Part model, mm, in its own coordinate system. Face numbers are marked on the shaded views. A direction names the side the tool comes from. Round coordinates to 2 decimals unless told otherwise and drop trailing zeros. Loops run counter-clockwise (first coordinate to the right, second up) from the corner with the lowest first, then second, coordinate; pieces in that order, holes last. Notation, with made-up numbers: (-5, 62) -> (9, 62) arc R15 cw to (9, 83) -> close; hole circle Ø3 at (-19.5, 45). An arc over 180 degrees is marked (long way). Answer as CSV lines item,"result".
from build123d import *

# Parameters (mm, degrees)
F0_W     = 205
F0_H     = 236
F0_R     = 2.25
F0_W_2   = 51
F0_H_2   = 216
F1_DEPTH = 25
F2_W     = 18
F2_H     = 18
F3_DEPTH = 10
F4_R     = 6
F5_DEPTH = 23


with BuildPart() as f1:
    # F0 (on Top) → F1 (new body)
    with BuildSketch(Plane.XY):
        Rectangle(F0_W, F0_H)
        with Locations((-33.5, -54)):
            Circle(F0_R, mode=Mode.SUBTRACT)
        with Locations((33.5, -54)):
            Circle(F0_R, mode=Mode.SUBTRACT)
        with Locations((-67, 0)):
            Rectangle(F0_W_2, F0_H_2, mode=Mode.SUBTRACT)
        with Locations((-33.5, 54)):
            Circle(F0_R, mode=Mode.SUBTRACT)
        Rectangle(F0_W_2, F0_H_2, mode=Mode.SUBTRACT)
        with Locations((33.5, 54)):
            Circle(F0_R, mode=Mode.SUBTRACT)
        with Locations((67, 0)):
            Rectangle(F0_W_2, F0_H_2, mode=Mode.SUBTRACT)
    extrude(amount=F1_DEPTH)

    # F2 (on face) → F3 (cut, through all)
    with BuildSketch(Plane.XZ.offset(118)):
        with Locations((-73.5, 16)):
            Rectangle(F2_W, F2_H)
        with Locations((-6.5, 16)):
            Rectangle(F2_W, F2_H)
        with Locations((60.5, 16)):
            Rectangle(F2_W, F2_H)
    extrude(amount=-F3_DEPTH, mode=Mode.SUBTRACT)

    # F4 (on face) → F5 (cut)
    with BuildSketch(Plane.XY.offset(25)):
        with Locations((-33.5, 54)):
            Circle(F4_R)
        with Locations((-33.5, -54)):
            Circle(F4_R)
        with Locations((33.5, 54)):
            Circle(F4_R)
        with Locations((33.5, -54)):
            Circle(F4_R)
    extrude(amount=-F5_DEPTH, mode=Mode.SUBTRACT)


solid = f1.part
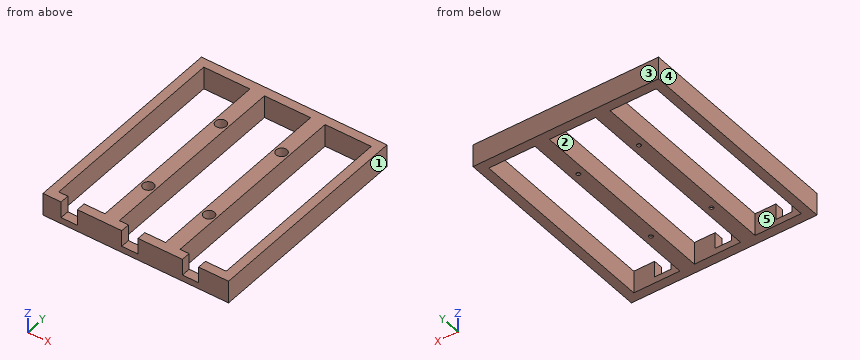
Q1. Saw through at B-B, the plane y = -94. Write the cut outline in (x, z), then the cut area to 3 significant figures.
Geometry results:
outline,"(-102.5, 0) -> (-92.5, 0) -> (-92.5, 25) -> (-102.5, 25) -> close; (-41.5, 0) -> (-25.5, 0) -> (-25.5, 25) -> (-41.5, 25) -> close; (25.5, 0) -> (41.5, 0) -> (41.5, 25) -> (25.5, 25) -> close; (92.5, 0) -> (102.5, 0) -> (102.5, 25) -> (92.5, 25) -> close"
area,"1,300 mm2"
Q2. Saw through at C-C, the plane z = 21.25. Give the number of separate pieces and of enclosed holes in the cut face, then the cut area to 3 significant figures.
Geometry results:
separate pieces,"1"
enclosed holes,"4"
area,"14,300 mm2"
Q3. Two-plate mould, pull along X, no slides. Class the marked faces 1, 2 and 3: pulls with the +X half, pulls with the -X half, needs draft (parallel to the pull), parting line crosses it, or undercut.
Geometry results:
face 1,"pulls with the +X half"
face 2,"undercut"
face 3,"needs draft"
Q4. Which spindle directions (+Z, -Z, +X, -X, +Y, -Y) get a long thin tool onto all of the face, cutting with end or side? Do the marked faces 4 and 5. Say none if no direction does.
Geometry results:
face 4,"+Z, -Z, -X, +Y, -Y"
face 5,"+Z, -Z"
Q5. Saw through at D-D, the plane x = -73. Write the cut outline in (y, z).
Geometry results:
outline,"(-118, 0) -> (-108, 0) -> (-108, 7) -> (-118, 7) -> close; (108, 0) -> (118, 0) -> (118, 25) -> (108, 25) -> close"
Q6. Drop flat-ended pins along their axis: P1, Ø3.5, axis at x = 33.5, y = 54, coming from the +Z side; P2, Ø3.5, axis at x = -33.5, y = 51.5, coming from the +Z side; P3, Ø8, axis at x = -74, y = -115, coming from the +Z side. Give the stop position or say it passes through.
Geometry results:
P1,"through"
P2,"z = 2"
P3,"z = 7"
Q7. Drill centre lines: line 1 along Y through (x, z) = (-33.5, 1.45); line 2 along X through (y, z) = (-54, 0.9); line 3 along X through (y, z) = (-13.5, 13.75). Where is each one in solid material? Low to high.
Geometry results:
line 1,"-118 to -56.25, -51.75 to 51.75, 56.25 to 118"
line 2,"-102.5 to -92.5, -41.5 to -35.75, -31.25 to -25.5, 25.5 to 31.25, 35.75 to 41.5, 92.5 to 102.5"
line 3,"-102.5 to -92.5, -41.5 to -25.5, 25.5 to 41.5, 92.5 to 102.5"
Q8. Saw through at A-A, the plane x = 81. Write the cut outline in (y, z), then the cut area to 3 significant figures.
Geometry results:
outline,"(-118, 0) -> (-108, 0) -> (-108, 25) -> (-118, 25) -> close; (108, 0) -> (118, 0) -> (118, 25) -> (108, 25) -> close"
area,"500 mm2"
